Check sheet for the modelled part. Datum: model origin and axes. Units: mm. A direction names the side the tool comes from. Coordinates: 2 decimals unless noted, no trailing zeros. Loops run counter-clockwise (first coordinate to the right, second up) from the corner with the lowest first, then second, coordinate; pieces in that order, holes last. Notation, with made-up numbers: M 84,-20.5 L 111,-20.5 A8 cw 111,-8.5 Z; hole C 15.25,46.25 d9. An arc over 180 degrees is marked long. Answer as CSV lines item,"result". Start each with the question number.
Autodesk Inventor part; units mm, degrees
ref_plane "YZ Plane" through (0, 0, 0) normal (1, 0, 0) x (0, 1, 0)
ref_plane "XZ Plane" through (0, 0, 0) normal (0, 1, 0) x (-1, 0, 0)
ref_plane "XY Plane" through (0, 0, 0) normal (0, 0, 1) x (1, 0, 0)
sketch "Sketch1" plane through (0, 0, 0) normal (0, 0, 1) x (1, 0, 0)
  circle A0 centre (0, 0) radius 2.5
  dimension "d0" = 5
extrude "Extrusion1" add sketch "Sketch1" along normal blind 10
thread "Thread1"
sketch "Sketch2" plane through (0, 0, 0) normal (0, 1, 0) x (-1, 0, 0)
  line L0 (0, 10.0728) -> (-4.75, 10.0728)
  line L1 (2.5, 10) -> (-2.5, 10)
  line L2 (0, 10) -> (-4.75, 10)
  line L3 (0, 10) -> (0, 12.75)
  line L4 (0, 12.75) -> (-2.85, 12.75)
  arc A0 (-2.85, 12.75) -> (-4.75, 10) centre (-1.457, 9.7562) ccw
  point P0 (0, 0)
  dimension "d5" = 4.75
  dimension "d6" = 2.75
  dimension "d7" = 2.85
  dimension "d8" = 3.302
revolve "Revolution1" add sketch "Sketch2" angle 360 about axis through (0, 0, 10) along (0, 0, 1)
sketch "Sketch3" plane through (0, 0, 12.75) normal (0, 0, 1) x (1, 0, 0)
  circle A0 centre (0, 0) radius 2.5
  line L0 (0, 2.5) -> (2.1651, 1.25)
  line L1 (2.1651, 1.25) -> (2.1651, -1.25)
  line L2 (2.1651, -1.25) -> (0, -2.5)
  line L3 (0, -2.5) -> (-2.1651, -1.25)
  line L4 (-2.1651, -1.25) -> (-2.1651, 1.25)
  line L5 (-2.1651, 1.25) -> (0, 2.5)
extrude "Extrusion2" cut sketch "Sketch3" against normal blind 1.56 contours L1 L2 L3 L4 L5 L0
properties part number "5mm Button Head Screw Botch"
Item 1: Sectioned sample at A-A, the plane z = 3.5. Record the boundary of the cut face in (x, y), and give its area (3 significant figures).
Item 2: Go/stop test with flat-tipped pins: pin 1 (3 mm diameter, centred on x = -1.5, z = 7.5, fed in from +Y); pin 2 (1.7 mm diameter, centred on y = 0, z = 11.5, fed in from +X); pin 3 (1.7 mm diameter, centred on y = 0.5, z = 12, fed in from -X). Record where each tip stops, or that it passes through.
Item 3: Release check for a two-part mould opening along Y. For faces 1 (the face through (-0.54, 2.44, 4.93)), 2 (the face through (0, 0, 0)), 3 (the face through (1.07, 1.88, 11.98)) record: released by +Y, released by -Y, zero draft, split by the parting line, or undercut.
Item 4: Set-up check for faces 4 (the face through (2, -2, 10)), 5 (the face through (2.165, 0, 12)): record each of +Z, -Z, +X, -X, +Y, -Y from which the full face is reachable in a straight line by a thin tool's end or side.
Item 5: Material ranges on line 1 (Y direction, x = 0.75, z = 12); line 2 (Z direction, x = 0.25, y = -0.5); line 3 (Z direction, x = 3.25, y = 0.5), recorded low to high. Write a range as from..to.
Reply:
1,outline,"C 0,0 d5"
1,area,"19.6 mm²"
2,pin 1,"y = 2.5"
2,pin 2,"x = 4.64"
2,pin 3,"x = -4.43"
3,face 1,"split by the parting line"
3,face 2,"zero draft"
3,face 3,"undercut"
4,face 4,"-Z"
4,face 5,"+Z"
5,line 1,"-3.81..-2.07, 2.07..3.81"
5,line 2,"0..11.19"
5,line 3,"10..12.5"
